```python
from build123d import *

# Parameters (mm, degrees)
CYLINDER001_R       = 3
CYLINDER001_DEPTH   = 10
CYLINDER_R          = 15
CYLINDER_DEPTH      = 27
CYLINDER_ROLL_ANGLE = 15.99999
BOX002_W            = 20
BOX002_H            = 10
BOX002_DEPTH        = 25
BOX004_W            = 3
BOX004_H            = 3
BOX004_DEPTH        = 3
BOX003_W            = 43
BOX003_H            = 15
BOX003_DEPTH        = 3
BOX001_W            = 10
BOX001_H            = 30
BOX001_DEPTH        = 10
BOX_W               = 20
BOX_H               = 45
BOX_DEPTH           = 3
FILLET_R            = 5
FILLET001_R         = 3
FILLET002_R         = 3
FILLET003_R         = 1
FILLET004_R         = 1
FILLET005_R         = 1
FILLET006_R         = 1


with BuildPart() as cylinder001:
    # Cylinder001 → Cylinder001 (new body)
    with BuildSketch(Plane(origin=(23, 8, -1), x_dir=(1, 0, 0), z_dir=(0, 0, 1))):
        Circle(CYLINDER001_R)
    extrude(amount=CYLINDER001_DEPTH)


with BuildPart() as cylinder:
    # Cylinder → Cylinder (new body)
    with BuildSketch(Plane.XY):
        Circle(CYLINDER_R)
    extrude(amount=CYLINDER_DEPTH)


with BuildPart() as cylinder_1:
    # Cylinder roll: moved
    add(cylinder.part.rotate(Axis((0, 0, 0), (1, 0, 0)), CYLINDER_ROLL_ANGLE))


with BuildPart() as cylinder_2:
    # Cylinder placement: moved
    add(cylinder_1.part.moved(Location((30, 13, 7))))


with BuildPart() as prise:
    # Box002 → Box002 (new body)
    with BuildSketch(Plane(origin=(20, -10, 0), x_dir=(1, 0, 0), z_dir=(0, 0, 1))):
        with Locations((10, 5)):
            Rectangle(BOX002_W, BOX002_H)
    extrude(amount=BOX002_DEPTH)

    # Cut001: cut Cylinder
    add(cylinder_2.part, mode=Mode.SUBTRACT)


with BuildPart() as prise_1:
    # Cut001 placement: moved
    add(prise.part.moved(Location((3, 0, 0))))


with BuildPart() as obj1:
    # Box004 → Box004 (new body)
    with BuildSketch(Plane(origin=(20, 5, 0), x_dir=(1, 0, 0), z_dir=(0, 0, 1))):
        with Locations((1.5, 1.5)):
            Rectangle(BOX004_W, BOX004_H)
    extrude(amount=BOX004_DEPTH)


with BuildPart() as extension_plan:
    # Box003 → Box003 (new body)
    with BuildSketch(Plane(origin=(0, -10, 0), x_dir=(1, 0, 0), z_dir=(0, 0, 1))):
        with Locations((21.5, 7.5)):
            Rectangle(BOX003_W, BOX003_H)
    extrude(amount=BOX003_DEPTH)


with BuildPart() as box02:
    # Box001 → Box001 (new body)
    with BuildSketch(Plane(origin=(5, 20, -3), x_dir=(1, 0, 0), z_dir=(0, 0, 1))):
        with Locations((5, 15)):
            Rectangle(BOX001_W, BOX001_H)
    extrude(amount=BOX001_DEPTH)


with BuildPart() as cut002:
    # Box → Box (new body)
    with BuildSketch(Plane.XY):
        with Locations((10, 22.5)):
            Rectangle(BOX_W, BOX_H)
    extrude(amount=BOX_DEPTH)

    # Cut: cut Box02
    add(box02.part, mode=Mode.SUBTRACT)

    # Fusion: union Extension plan
    add(extension_plan.part)

    # Fusion001: union obj1
    add(obj1.part)

    # Fusion002: union Prise
    add(prise_1.part)

    # Fillet
    fillet_edges = [cut002.edges().sort_by_distance(p)[0] for p in [
        (0, -10, 1.5),
    ]]
    fillet(fillet_edges, radius=FILLET_R)

    # Fillet001
    fillet001_edges = [cut002.edges().sort_by_distance(p)[0] for p in [
        (43, 5, 1.5),
    ]]
    fillet(fillet001_edges, radius=FILLET001_R)

    # Fillet002
    fillet002_edges = [cut002.edges().sort_by_distance(p)[0] for p in [
        (43, -10, 14),
    ]]
    fillet(fillet002_edges, radius=FILLET002_R)

    # Fillet003
    fillet003_edges = [cut002.edges().sort_by_distance(p)[0] for p in [
        (5, 45, 1.5),
    ]]
    fillet(fillet003_edges, radius=FILLET003_R)

    # Fillet004
    fillet004_edges = [cut002.edges().sort_by_distance(p)[0] for p in [
        (20, 45, 1.5),
    ]]
    fillet(fillet004_edges, radius=FILLET004_R)

    # Fillet005
    fillet005_edges = [cut002.edges().sort_by_distance(p)[0] for p in [
        (0, 45, 1.5),
    ]]
    fillet(fillet005_edges, radius=FILLET005_R)

    # Fillet006
    fillet006_edges = [cut002.edges().sort_by_distance(p)[0] for p in [
        (15, 45, 1.5),
    ]]
    fillet(fillet006_edges, radius=FILLET006_R)

    # Cut002: cut Cylinder001
    add(cylinder001.part, mode=Mode.SUBTRACT)


solid = cut002.part
```
Input: part model. Units: mm. Frame: model coordinates. A direction names the side the tool comes from. Give positions to 0.01 mm unless a question says otherwise; leave off trailing zeros. Write each loop counter-clockwise with the first axis right and the second up, starting at its lowest first coordinate (ties: lowest second). Pieces come first, ordered by that corner, then holes. Notation, with made-up numbers: (46, 16) - (71, 16) arc R12 cw to (71, 28) - close; hole circle Ø3 at (76.25, 5.5). An arc over 180 degrees is marked (long way). Write item = value, one per line. Start each with the question number.
1) Cut plane A-A (y = 39). Return loops of the section in (x, z), and give its area (3 significant figures).
2) Material intervals for L1, parallel to X at y = 22.5, z = 1.5; L2, parallel to Z at x = 17.5, y = 19; L3, parallel to Y at x = 23, z = 1.75, sorted ascending. Write a range as [from, to].
3) Draft query along X for faces 4 (the face through (31, 5, 1)), 5 (the face through (20, 26, 1)), 6 (the face through (5, 32, 1)). Return one class per face: pulls with the +X half, pulls with the -X half, needs draft (parallel to the pull), parting line crosses it, or undercut.
4) Cut plane D-D (x = 11.5). Return loops of the section in (y, z).
5) Reachability of faces 1 (the face through (23, -5, 14)), 2 (the face through (10, 20, 1)), 3 (the face through (16, 12, 0)) from +Z, -Z, +X, -X, +Y, -Y: full face, straight path, thin tool, end or side. Return the list, or none.
6) Cut plane C-C (y = 7). Return loops of the section in (x, z).
7) Cut plane B-B (x = 32). Return loops of the section in (y, z), and give its area (3 significant figures).
8) Pin query (flat end, axial travel): pin 1 (0.9 mm diameter, centred on x = 10, z = 1, fed in from +Y); pin 2 (1.5 mm diameter, centred on y = -1, z = 15, fed in from -X); pin 3 (1.5 mm diameter, centred on x = 35.5, z = 6.5, fed in from +Y); pin 4 (6 mm diameter, centred on x = 6, y = 0, fed in from -Z). Return the tip coordinate at first contact, or that it passes through.
Answers follow:
q1.outline = (0, 0) - (5, 0) - (5, 3) - (0, 3) - close; (15, 0) - (20, 0) - (20, 3) - (15, 3) - close
q1.area = 30.0 mm^2
q2.L1 = [0, 5], [15, 20]
q2.L2 = [0, 3]
q2.L3 = [-10, 5]
q3.face_4 = needs draft
q3.face_5 = pulls with the +X half
q3.face_6 = undercut
q4.outline = (-10, 0) - (20, 0) - (20, 3) - (-10, 3) - close
q5.face_1 = +Z, -X, +Y, -Y
q5.face_2 = +Z, -Z, +Y
q5.face_3 = -Z, +X, -X, +Y, -Y
q6.outline = (0, 0) - (20.17, 0) - (20.17, 3) - (0, 3) - close
q7.outline = (-10, 0) - (5, 0) - (5, 3) - (0, 3) - (0, 3.27) - (-0.95, 3) - (-1.42, 3) - (-7.73, 25) - (-10, 25) - close
q7.area = 164 mm^2
q8.pin_1 = 20
q8.pin_2 = 23
q8.pin_3 = -1.98
q8.pin_4 = 0
